Build history of the part. All positions in model axes, mm. A direction names the side the tool comes from. Give positions to 0.01 mm unless a question says otherwise; leave off trailing zeros. Order: outer loops, then holes, each group sorted by start corner. A loop starts at its lowest first (then second) coordinate and runs counter-clockwise, first axis right, second up. Notation, with made-up numbers: (-5.75, -28) -> (42.25, -28) arc R25 cw to (42.25, -11) -> close; hole circle Ø10 at (18, 23). An arc over 180 degrees is marked (long way). One line per question, with ' | ' between items. Start each with the question number.
(1) Cut at B-B (y = -13). Give the cut face in (x, z), then the cut area to 3 significant figures.
(2) Cut at C-C (z = 23.5). Give the cut face in (x, y), then the cut area to 3 significant figures.
(3) Drill centre lines: L1, parallel to Y at x = 0, z = 68.75; L2, parallel to Y at x = 0, z = 10; L3, parallel to Z at x = -5, y = 12. Where is each one in solid material? Low to high. Write a range as from..to.
(4) Pull direction Y, two halves, no side cores. Call faces 1 (the face through (-0.325, -14.464, 68.521)), 2 (the face through (-1.73, -7.81, 31.87)), 3 (the face through (0, 0, 70)), 4 (the face through (-0.325, 11.536, 68.521)): +Y half, -Y half, draft (parallel to the pull), parting line (faces both ways), or undercut.
(5) Cut at A-A (x = 11). Give the cut face in (y, z).
(6) Pin check, flat tips, straight feed: pin 1 Ø10 at (x, y) = (3.5, 6.5) entering from -Z; pin 2 Ø4 at (x, z) = (-0.5, 43.5) entering from -Y; pin 3 Ø10 at (y, z) = (3, 10) entering from -X; pin 4 Ø5 at (y, z) = (-9.5, 54) entering from -X. Stop position of each tip, or through.
(7) Cut at D-D (y = 6.5). Give the number of separate pieces and of enclosed holes in the cut face, then the cut area to 3 significant figures.
(8) Which spindle directions (+Z, -Z, +X, -X, +Y, -Y) get a long thin tool onto all of the face, cutting with end or side? Do faces 5 (the face through (7, -7, 67)), 6 (the face through (-10.566, 5.169, 68.521)). Say none if no direction does.
from build123d import *

# Parameters (mm, degrees)
CROQUIS1_R              = 8
SALIENTE_EXTRUIR1_DEPTH = 67
CROQUIS2_R              = 17
SALIENTE_EXTRUIR2_DEPTH = 3
CROQUIS3_R              = 9
SALIENTE_EXTRUIR3_DEPTH = 5
SALIENTE_EXTRUIR3_TAPER = 23
CROQUIS4_R              = 1.5
CORTAR_EXTRUIR2_DEPTH   = 5


with BuildPart() as part:
    # Croquis1 → Saliente-Extruir1 (new body)
    with BuildSketch(Plane.XY):
        Circle(CROQUIS1_R)
    extrude(amount=SALIENTE_EXTRUIR1_DEPTH)

    # Croquis2 → Saliente-Extruir2 (add)
    with BuildSketch(Plane.XY.offset(67)):
        Circle(CROQUIS2_R)
    extrude(amount=SALIENTE_EXTRUIR2_DEPTH)

    # Croquis3 → Saliente-Extruir3 (add)
    with BuildSketch(Plane(origin=(0, 0, 67), x_dir=(-1, 0, 0), z_dir=(0, 0, -1))):
        Circle(CROQUIS3_R)
    extrude(amount=SALIENTE_EXTRUIR3_DEPTH, taper=SALIENTE_EXTRUIR3_TAPER)

    # Croquis4 → Cortar-Extruir2 (cut)
    with BuildSketch(Plane.XY.offset(70)):
        with Locations((0, 13)):
            Circle(CROQUIS4_R)
        with Locations((11.258330249, 6.5)):
            Circle(CROQUIS4_R)
        with Locations((11.258330249, -6.5)):
            Circle(CROQUIS4_R)
        with Locations((0, -13)):
            Circle(CROQUIS4_R)
        with Locations((-11.258330249, -6.5)):
            Circle(CROQUIS4_R)
        with Locations((-11.258330249, 6.5)):
            Circle(CROQUIS4_R)
    extrude(amount=-CORTAR_EXTRUIR2_DEPTH, mode=Mode.SUBTRACT)


solid = part.part
Result set:
1) outline: (-10.95, 67) -> (-1.5, 67) -> (-1.5, 70) -> (-10.95, 70) -> close; (1.5, 67) -> (10.95, 67) -> (10.95, 70) -> (1.5, 70) -> close | area: 56.7 mm2
2) outline: circle Ø16 at (0, 0) | area: 201 mm2
3) L1: y = -17..-14.5, -11.5..11.5, 14.5..17 | L2: y = -8..8 | L3: z = 67..70
4) face 1: undercut | face 2: parting line | face 3: draft | face 4: undercut
5) outline: (-12.96, 67) -> (-7.98, 67) -> (-7.98, 70) -> (-12.96, 70) -> close; (-5.02, 67) -> (5.02, 67) -> (5.02, 70) -> (-5.02, 70) -> close; (7.98, 67) -> (12.96, 67) -> (12.96, 70) -> (7.98, 70) -> close
6) pin 1: stops at z = 0 | pin 2: stops at y = -8 | pin 3: stops at x = -8 | pin 4: stops at x = -3.87
7) separate pieces: 3 | enclosed holes: 0 | area: 705 mm2
8) face 5: -Z | face 6: +Z, -Z
